Design review of the part built by this model. Coordinates are the model's own, in mm. A direction names the side the tool comes from. Give positions to 0.01 mm unless a question says otherwise; leave off trailing zeros. Loops run counter-clockwise (first coordinate to the right, second up) from the corner with the lowest first, then second, coordinate; pieces in that order, holes last. Notation, with made-up numbers: M 84.5,17.5 L 124.5,17.5 A16 ccw 124.5,40.5 Z; hole C 35,-17 d10. An arc over 180 degrees is marked long. Use a Markdown table: item, result. Add a question column.
(1) Add section C-C, the plane z = 0.4. Give the boundary of the cut face in (x, y).
(2) For faces 4 (the face through (5, 0, 0)), 5 (the face through (-3, 0, 2)), 6 (the face through (0, 0, 4)), list the 3-axis set-ups (+Z, -Z, +X, -X, +Y, -Y) from which the entire face can be reached by the end or side of a thin tool; tool diameter is ignored.
(3) Add section A-A, the plane y = 1.25. Give the boundary of the cut face in (x, z).
(4) Add section B-B, the plane x = -2. Give the boundary of the cut face in (y, z).
(5) Draft analysis for pull direction X (two halves, no side actions). For faces 1 (the face through (9.46, 2.45, 0.49)), 2 (the face through (18, 0, 6)), 3 (the face through (18.477, 0.15, 3.465)), state which applies: pulls with the +X half, pulls with the -X half, needs draft (parallel to the pull), parting line crosses it, or undercut.
(6) Insertion check: pin 1 Ø1.8 at (x, y) = (-1, -0.5) entering from +Z; pin 2 Ø3 at (y, z) = (2, 1) entering from +X; pin 3 Ø1 at (x, z) = (0, 4) entering from +Y. Each pin has a flat end and moves straight along its axis. Give the tip position at first contact, or say it passes through.
(7) For probe 1 along Z at (x, y) = (0, 1.5); probe 2 along Z at (x, y) = (5.25, 2); probe 3 along X at (y, z) = (0.25, 2.85), list the stretches that pass through material, from the lowest coordinate up.
(8) Add section D-D, the plane y = -0.25. Give the boundary of the cut face in (x, z).
```python
from build123d import *

# Parameters (mm, degrees)
BOSS_EXTRUDE1_DEPTH = 1
SKETCH2_R           = 0.5
SKETCH2_R_2         = 3
BOSS_EXTRUDE2_DEPTH = 3
SKETCH3_R           = 0.5
BOSS_EXTRUDE3_DEPTH = 2


with BuildPart() as part:
    # Sketch1 → Boss-Extrude1 (new body)
    with BuildSketch(Plane.XY):
        with BuildLine():
            Line((18, 1), (0.669804359, 3.943521538))
            ThreePointArc((0.669804359, 3.943521538), (-3.985855376, 0.336090648), (0, -4))
            Line((0, -4), (18, -1))
            ThreePointArc((18, -1), (19, 0), (18, 1))
        make_face()
    extrude(amount=BOSS_EXTRUDE1_DEPTH)

    # Sketch2 → Boss-Extrude2 (add)
    with BuildSketch(Plane.XY.offset(1)):
        with Locations((18, 0)):
            Circle(SKETCH2_R)
        Circle(SKETCH2_R_2)
    extrude(amount=BOSS_EXTRUDE2_DEPTH)

    # Sketch3 → Boss-Extrude3 (add)
    with BuildSketch(Plane.XY.offset(4)):
        with Locations((18, 0)):
            Circle(SKETCH3_R)
    extrude(amount=BOSS_EXTRUDE3_DEPTH)


solid = part.part
```
Established:
| question | item | result |
|---|---|---|
| 1 | outline | M 0,-4 L 18,-1 A1 ccw 18,1 L 0.67,3.94 A4 ccw long Z |
| 2 | face 4 | -Z, +X, -X, +Y, -Y |
| 2 | face 5 | +Z |
| 2 | face 6 | +Z, -X, +Y, -Y |
| 3 | outline | M -3.8,0 L 16.53,0 L 16.53,1 L 2.73,1 L 2.73,4 L -2.73,4 L -2.73,1 L -3.8,1 Z |
| 4 | outline | M -3.46,0 L 3.46,0 L 3.46,1 L 2.24,1 L 2.24,4 L -2.24,4 L -2.24,1 L -3.46,1 Z |
| 5 | face 1 | pulls with the +X half |
| 5 | face 2 | needs draft |
| 5 | face 3 | undercut |
| 6 | pin 1 | z = 4 |
| 6 | pin 2 | x = 18.87 |
| 6 | pin 3 | y = 3 |
| 7 | probe 1 | 0 to 4 |
| 7 | probe 2 | 0 to 1 |
| 7 | probe 3 | -2.99 to 2.99, 17.57 to 18.43 |
| 8 | outline | M -3.99,0 L 18.97,0 L 18.97,1 L 18.43,1 L 18.43,6 L 17.57,6 L 17.57,1 L 2.99,1 L 2.99,4 L -2.99,4 L -2.99,1 L -3.99,1 Z |
